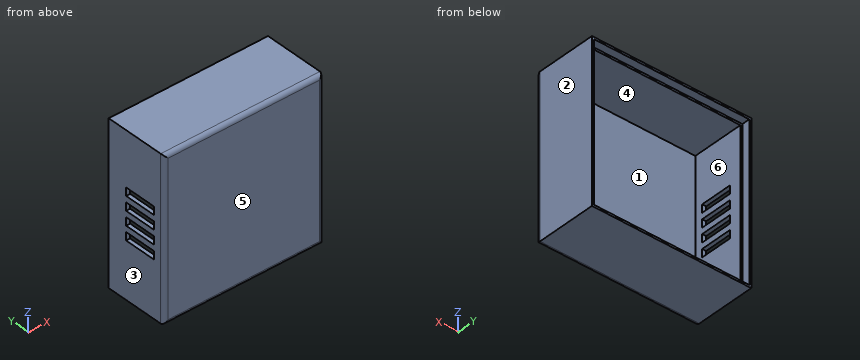
from build123d import *

# Parameters (mm, degrees)
SKETCH_1_W          = 40
SKETCH_1_H          = 40
EXTRUDE_1_DEPTH     = 16
SKETCH_2_W          = 38
SKETCH_2_H          = 38
CUT_EXTRUDE_2_DEPTH = 15
FILLET_2_R          = 1
SKETCH_5_W          = 38
SKETCH_5_H          = 2
CUT_EXTRUDE_4_DEPTH = 0.5
SKETCH_6_W          = 38.5
SKETCH_6_H          = 2
CUT_EXTRUDE_5_DEPTH = 0.5
SKETCH_7_W          = 38.5
SKETCH_7_H          = 2
CUT_EXTRUDE_6_DEPTH = 0.5
SKETCH_8_W          = 39
SKETCH_8_H          = 2
CUT_EXTRUDE_7_DEPTH = 0.5
SKETCH_9_W          = 2
SKETCH_9_H          = 8
CUT_EXTRUDE_9_DEPTH = 10


with BuildPart() as part:
    # Эскиз1 → Бобышка-Вытянуть1 (new body)
    with BuildSketch(Plane(origin=(0, 0, 0), x_dir=(1, 0, 0), z_dir=(0, 1, 0))):
        with Locations((18.915, -19.461)):
            Rectangle(SKETCH_1_W, SKETCH_1_H)
    extrude(amount=EXTRUDE_1_DEPTH)

    # Эскиз2 → Вырез-Вытянуть2 (cut)
    with BuildSketch(Plane(origin=(0, 16, 0), x_dir=(1, 0, 0), z_dir=(0, 1, 0))):
        with Locations((18.915, -19.461)):
            Rectangle(SKETCH_2_W, SKETCH_2_H)
    extrude(amount=-CUT_EXTRUDE_2_DEPTH, mode=Mode.SUBTRACT)

    # Скругление2
    fillet_2_edges = [part.edges().sort_by_distance(p)[0] for p in [
        (18.915, 0, -0.539),
        (38.915, 0, 19.461),
        (18.915, 0, 39.461),
        (-1.085, 0, 19.461),
    ]]
    fillet(fillet_2_edges, radius=FILLET_2_R)

    # Эскиз5 → Вырез-Вытянуть4 (cut)
    with BuildSketch(Plane(origin=(0, 0, 38.461), x_dir=(-1, 0, 0), z_dir=(0, 0, -1))):
        with Locations((-18.915, 15)):
            Rectangle(SKETCH_5_W, SKETCH_5_H)
    extrude(amount=-CUT_EXTRUDE_4_DEPTH, mode=Mode.SUBTRACT)

    # Эскиз6 → Вырез-Вытянуть5 (cut)
    with BuildSketch(Plane(origin=(-0.085, 0, 0), x_dir=(0, 0, -1), z_dir=(1, 0, 0))):
        with Locations((-19.711, 15)):
            Rectangle(SKETCH_6_W, SKETCH_6_H)
    extrude(amount=-CUT_EXTRUDE_5_DEPTH, mode=Mode.SUBTRACT)

    # Эскиз7 → Вырез-Вытянуть6 (cut)
    with BuildSketch(Plane.XY.offset(0.461)):
        with Locations((18.665, 15)):
            Rectangle(SKETCH_7_W, SKETCH_7_H)
    extrude(amount=-CUT_EXTRUDE_6_DEPTH, mode=Mode.SUBTRACT)

    # Эскиз8 → Вырез-Вытянуть7 (cut)
    with BuildSketch(Plane.ZY.offset(-37.915)):
        with Locations((19.461, 15)):
            Rectangle(SKETCH_8_W, SKETCH_8_H)
    extrude(amount=-CUT_EXTRUDE_7_DEPTH, mode=Mode.SUBTRACT)

    # Эскиз9 → Вырез-Вытянуть9 (cut)
    with BuildSketch(Plane.ZY.offset(1.085)):
        with Locations((17.961, 6.970991383)):
            Rectangle(SKETCH_9_W, SKETCH_9_H)
        with Locations((14.461, 6.970991383)):
            Rectangle(SKETCH_9_W, SKETCH_9_H)
        with Locations((21.461, 6.970991383)):
            Rectangle(SKETCH_9_W, SKETCH_9_H)
        with Locations((24.961, 6.970991383)):
            Rectangle(SKETCH_9_W, SKETCH_9_H)
    extrude(amount=-CUT_EXTRUDE_9_DEPTH, mode=Mode.SUBTRACT)


solid = part.part
Part model, mm, in its own coordinate system. Face numbers are marked on the shaded views. A direction names the side the tool comes from. Give positions to 0.01 mm unless a question says otherwise; leave off trailing zeros. Loops run counter-clockwise (first coordinate to the right, second up) from the corner with the lowest first, then second, coordinate; pieces in that order, holes last.
(1) Band-saw the part on A-A (y = 8.5). Write the cut outline in (x, z) (3 decimals), and give its area (3 significant figures).
Return value:
outline: (-1.085, -0.539) - (38.915, -0.539) - (38.915, 39.461) - (-1.085, 39.461) - (-1.085, 25.961) - (-0.085, 25.961) - (-0.085, 38.461) - (37.915, 38.461) - (37.915, 0.461) - (-0.085, 0.461) - (-0.085, 13.461) - (-1.085, 13.461) - close; (-1.085, 15.461) - (-0.085, 15.461) - (-0.085, 16.961) - (-1.085, 16.961) - close; (-1.085, 18.961) - (-0.085, 18.961) - (-0.085, 20.461) - (-1.085, 20.461) - close; (-1.085, 22.461) - (-0.085, 22.461) - (-0.085, 23.961) - (-1.085, 23.961) - close
area: 148 mm2
(2) Band-saw the part on B-B (z = 18). Write the cut outline in (x, y) (3 decimals).
Return value:
outline: (-1.085, 1) arc R1 ccw to (-0.085, 0) - (37.915, 0) arc R1 ccw to (38.915, 1) - (38.915, 16) - (38.415, 16) - (38.415, 14) - (37.915, 14) - (37.915, 1) - (-0.085, 1) - (-0.085, 2.971) - (-1.085, 2.971) - close; (-1.085, 10.971) - (-0.085, 10.971) - (-0.085, 14) - (-0.585, 14) - (-0.585, 16) - (-1.085, 16) - close
(3) 3-axis set-ups, long thin cutter, end or side, ignore diameter. For the marked faces 5 and 6: which of +Z, -Z, +X, -X, +Y, -Y reach the whole face in a straight line?
Return value:
face 5: +Z, -Z, +X, -X, -Y
face 6: +Y
(4) Band-saw the part on D-D (z = 3). Write the cut outline in (x, y) (3 decimals).
Return value:
outline: (-1.085, 1) arc R1 ccw to (-0.085, 0) - (37.915, 0) arc R1 ccw to (38.915, 1) - (38.915, 16) - (38.415, 16) - (38.415, 14) - (37.915, 14) - (37.915, 1) - (-0.085, 1) - (-0.085, 14) - (-0.585, 14) - (-0.585, 16) - (-1.085, 16) - close
(5) Pin check, flat tips, straight feed: pin 1 (8 mm diameter, centred on x = 26, z = 16.5, fed in from +Y); pin 2 (0.5 mm diameter, centred on x = -0.5, z = 21, fed in from -Y). Stop position of each tip, or through.
Return value:
pin 1: stops at y = 1
pin 2: stops at y = 0.01
(6) Pull direction X, two halves, no side cores. Call the marked faces 1, 2, 3 and 4: pulls with the +X half, pulls with the -X half, needs draft (parallel to the pull), parting line crosses it, or undercut.
Return value:
face 1: undercut
face 2: pulls with the +X half
face 3: pulls with the -X half
face 4: undercut
(7) Band-saw the part on C-C (x = 6.5). Write the cut outline in (y, z), and give its area (3 significant figures).
Return value:
outline: (0, 0.46) arc R1 ccw to (1, -0.54) - (16, -0.54) - (16, -0.04) - (14, -0.04) - (14, 0.46) - (1, 0.46) - (1, 38.46) - (14, 38.46) - (14, 38.96) - (16, 38.96) - (16, 39.46) - (1, 39.46) arc R1 ccw to (0, 38.46) - close
area: 67.6 mm2
(8) Drill centre lines: line 1 along X through (y, z) = (4.75, 31) (3 decimals); line 2 along Z through (x, y) = (9.5, 11.25); line 3 along Z through (x, y) = (18, 15). Where is each one in solid material? Low to high.
Return value:
line 1: x = -1.085 to -0.085, 37.915 to 38.915
line 2: z = -0.54 to 0.46, 38.46 to 39.46
line 3: z = -0.54 to -0.04, 38.96 to 39.46
